from build123d import *

# Parameters (mm, degrees)
F1_W     = 2032
F1_H     = 558.8
F2_DEPTH = 19.05
F3_W     = 38.1
F3_H     = 38.1
F3_H_2   = 558.8
F4_DEPTH = 742.95


with BuildPart() as f2:
    # F1 (on offset) → F2 (new body)
    with BuildSketch(Plane.XY.offset(762)):
        with Locations((1016, 279.4)):
            Rectangle(F1_W, F1_H)
    extrude(amount=-F2_DEPTH)

    # F3 (on face) → F4 (join, through all)
    with BuildSketch(Plane(origin=(0, 0, 742.95), x_dir=(1, 0, 0), z_dir=(0, 0, -1))):
        with Locations((19.05, -19.05)):
            Rectangle(F3_W, F3_H)
        with Locations((19.05, -539.75)):
            Rectangle(F3_W, F3_H)
        with Locations((2012.95, -279.4)):
            Rectangle(F3_W, F3_H_2)
    extrude(amount=F4_DEPTH)


solid = f2.part
The listing builds one solid part. Answer for the finished solid, in the listing's coordinates (mm). A direction names the side the tool comes from. Coordinates: 2 decimals unless noted, no trailing zeros. Loops run counter-clockwise (first coordinate to the right, second up) from the corner with the lowest first, then second, coordinate; pieces in that order, holes last.
1) Flat-ended cylindrical pins translate along their axes: pin 1 Ø5 at (x, y) = (1814, 465) entering from -Z; pin 2 Ø8 at (y, z) = (486, 432.5) entering from -X. Find the tip coordinate at first contact, or state that the pin passes through.
2) Find section B-B on y = 101. Write down the section's boundary in (x, z), then the cut area to 3 significant figures.
3) Find section C-C on x = 1008. Write down the section's boundary in (y, z).
4) Determine the mould class of faces 4 (the face through (2032, 275, 386)), 5 (the face through (560, 0, 750)), 6 (the face through (38.1, 19, 377)) for opening direction X: pulls with the +X half, pulls with the -X half, needs draft (parallel to the pull), parting line crosses it, or undercut.
5) Find the intervals of material crossed by L1, parallel to Z at x = 344, y = 443; L2, parallel to X at y = 432.5, z = 339.5; L3, parallel to X at y = 28, z = 134.5, in increasing order.
6) Find section A-A on z = 259. Write down the section's boundary in (x, y), then the cut area to 3 significant figures.
7) A tool of negligible diameter and unlimited length cuts with its end or side. For faces 1 (the face through (19, 38.1, 377)), 2 (the face through (38.1, 540, 377)), 3 (the face through (19, 19, 0)), from which of +Z, -Z, +X, -X, +Y, -Y can it reach the whole face along a straight path? Write none if from no direction.
Values:
1. pin 1: stops at z = 742.95
1. pin 2: stops at x = 1993.9
2. outline: (0, 742.95) - (1993.9, 742.95) - (1993.9, 0) - (2032, 0) - (2032, 762) - (0, 762) - close
2. area: 67,000 mm2
3. outline: (0, 742.95) - (558.8, 742.95) - (558.8, 762) - (0, 762) - close
4. face 4: pulls with the +X half
4. face 5: needs draft
4. face 6: undercut
5. L1: z = 742.95 to 762
5. L2: x = 1993.9 to 2032
5. L3: x = 0 to 38.1, 1993.9 to 2032
6. outline: (0, 0) - (38.1, 0) - (38.1, 38.1) - (0, 38.1) - close; (0, 520.7) - (38.1, 520.7) - (38.1, 558.8) - (0, 558.8) - close; (1993.9, 0) - (2032, 0) - (2032, 558.8) - (1993.9, 558.8) - close
6. area: 24,200 mm2
7. face 1: -Z, -X
7. face 2: -Z, +Y, -Y
7. face 3: -Z, +X, -X, +Y, -Y
